from build123d import *

# Parameters (mm, degrees)
SKETCH1_W           = 119.2
SKETCH1_H           = 65.04
BOSS_EXTRUDE1_DEPTH = 2
SKETCH2_W           = 80
SKETCH2_H           = 2
SKETCH2_W_2         = 59.6
SKETCH2_H_2         = 2.5
BOSS_EXTRUDE2_DEPTH = 10
FILLET1_R           = 1
SKETCH3_W           = 80
SKETCH3_H           = 2
CUT_EXTRUDE1_DEPTH  = 7
SKETCH4_W           = 80
SKETCH4_H           = 2.5
SKETCH4_W_2         = 8
BOSS_EXTRUDE3_DEPTH = 10
FILLET2_R           = 1
FILLET3_R           = 1
CUT_EXTRUDE2_DEPTH  = 10
CUT_EXTRUDE3_DEPTH  = 10


with BuildPart() as part:
    # Sketch1 → Boss-Extrude1 (new body)
    with BuildSketch(Plane(origin=(0, 0, 0), x_dir=(1, 0, 0), z_dir=(0, 1, 0))):
        Rectangle(SKETCH1_W, SKETCH1_H)
    extrude(amount=BOSS_EXTRUDE1_DEPTH)

    # Sketch2 → Boss-Extrude2 (add)
    with BuildSketch(Plane(origin=(0, 2, 0), x_dir=(1, 0, 0), z_dir=(0, 1, 0))):
        with Locations((0, -9.48)):
            Rectangle(SKETCH2_W, SKETCH2_H)
        with Locations((0, -5.48)):
            Rectangle(SKETCH2_W, SKETCH2_H)
        with Locations((0, 28.27)):
            Rectangle(SKETCH2_W_2, SKETCH2_H_2)
    extrude(amount=BOSS_EXTRUDE2_DEPTH)

    # Fillet1
    fillet1_edges = [part.edges().sort_by_distance(p)[0] for p in [
        (40, 2, 9.48),
        (0, 2, 10.48),
        (-40, 2, 9.48),
        (40, 2, 5.48),
        (0, 2, 4.48),
        (-40, 2, 5.48),
        (-29.8, 2, -28.27),
        (29.8, 2, -28.27),
        (0, 2, -29.52),
    ]]
    fillet(fillet1_edges, radius=FILLET1_R)

    # Sketch3 → Cut-Extrude1 (cut)
    with BuildSketch(Plane(origin=(0, 12, 0), x_dir=(1, 0, 0), z_dir=(0, 1, 0))):
        with Locations((0, -5.48)):
            Rectangle(SKETCH3_W, SKETCH3_H)
        with Locations((0, -9.48)):
            Rectangle(SKETCH3_W, SKETCH3_H)
    extrude(amount=-CUT_EXTRUDE1_DEPTH, mode=Mode.SUBTRACT)

    # Sketch4 → Boss-Extrude3 (add)
    with BuildSketch(Plane(origin=(0, 2, 0), x_dir=(1, 0, 0), z_dir=(0, 1, 0))):
        with Locations((0, -28.77)):
            Rectangle(SKETCH4_W, SKETCH4_H)
        with Locations((52.6, -26.27)):
            Rectangle(SKETCH4_W_2, SKETCH4_H)
    boss_extrude3 = extrude(amount=BOSS_EXTRUDE3_DEPTH)

    # Fillet2
    fillet2_edges = [part.edges().sort_by_distance(p)[0] for p in [
        (-40, 2, 28.77),
        (48.6, 2, 26.27),
        (52.6, 2, 25.02),
        (40, 2, 28.77),
        (0, 2, 27.52),
    ]]
    fillet(fillet2_edges, radius=FILLET2_R)

    # Mirror1: Boss-Extrude3 across plane
    add(boss_extrude3.mirror(Plane.ZY))

    # Fillet3
    fillet3_edges = [part.edges().sort_by_distance(p)[0] for p in [
        (-48.6, 2, 26.27),
        (-52.6, 2, 25.02),
    ]]
    fillet(fillet3_edges, radius=FILLET3_R)

    # Sketch5 → Cut-Extrude2 (cut)
    with BuildSketch(Plane(origin=(0, 2, 0), x_dir=(1, 0, 0), z_dir=(0, 1, 0))):
        with BuildLine():
            Line((46.6, 22.52), (6.311514948, 22.52))
            Line((6.311514948, 22.52), (-46.6, 22.52))
            ThreePointArc((-46.6, 22.52), (-48.721320344, 21.641320344), (-49.6, 19.52))
            Line((-49.6, 19.52), (-49.6, 3.52))
            ThreePointArc((-49.6, 3.52), (-48.721320344, 1.398679656), (-46.6, 0.52))
            Line((-46.6, 0.52), (46.6, 0.52))
            ThreePointArc((46.6, 0.52), (48.721320344, 1.398679656), (49.6, 3.52))
            Line((49.6, 3.52), (49.6, 19.52))
            ThreePointArc((49.6, 19.52), (48.721320344, 21.641320344), (46.6, 22.52))
        make_face()
    extrude(amount=-CUT_EXTRUDE2_DEPTH, mode=Mode.SUBTRACT)

    # Sketch6 → Cut-Extrude3 (cut)
    with BuildSketch(Plane(origin=(0, 2, 0), x_dir=(1, 0, 0), z_dir=(0, 1, 0))):
        with BuildLine():
            Line((54.014213562, -5.94084617), (52.045315698, -3.971948306))
            ThreePointArc((52.045315698, -3.971948306), (51.396469, -3.538402803), (50.631102135, -3.386161868))
            Line((50.631102135, -3.386161868), (46.32782558, -3.386161868))
            ThreePointArc((46.32782558, -3.386161868), (44.913612017, -3.971948306), (44.32782558, -5.386161868))
            Line((44.32782558, -5.386161868), (44.32782558, -20.397912268))
            ThreePointArc((44.32782558, -20.397912268), (44.913612017, -21.812125831), (46.32782558, -22.397912268))
            Line((46.32782558, -22.397912268), (52.6, -22.397912268))
            ThreePointArc((52.6, -22.397912268), (54.014213562, -21.812125831), (54.6, -20.397912268))
            Line((54.6, -20.397912268), (54.6, -7.355059733))
            ThreePointArc((54.6, -7.355059733), (54.447759065, -6.589692868), (54.014213562, -5.94084617))
        make_face()
        with BuildLine():
            Line((39.82782558, -13.44932419), (24.210760832, -13.44932419))
            ThreePointArc((24.210760832, -13.44932419), (23.503654051, -13.742217409), (23.210760832, -14.44932419))
            Line((23.210760832, -14.44932419), (23.210760832, -23.393622011))
            ThreePointArc((23.210760832, -23.393622011), (23.650100661, -24.454282183), (24.710760832, -24.893622011))
            Line((24.710760832, -24.893622011), (39.32782558, -24.893622011))
            ThreePointArc((39.32782558, -24.893622011), (40.388485752, -24.454282183), (40.82782558, -23.393622011))
            Line((40.82782558, -23.393622011), (40.82782558, -14.44932419))
            ThreePointArc((40.82782558, -14.44932419), (40.534932361, -13.742217409), (39.82782558, -13.44932419))
        make_face()
        with BuildLine():
            Line((4.043952302, -24.893622011), (19.660852384, -24.893622011))
            ThreePointArc((19.660852384, -24.893622011), (20.367959165, -24.600728792), (20.660852384, -23.893622011))
            Line((20.660852384, -23.893622011), (20.660852384, -14.321364431))
            ThreePointArc((20.660852384, -14.321364431), (20.221512556, -13.260704259), (19.160852384, -12.821364431))
            Line((19.160852384, -12.821364431), (4.543952302, -12.821364431))
            ThreePointArc((4.543952302, -12.821364431), (3.48329213, -13.260704259), (3.043952302, -14.321364431))
            Line((3.043952302, -14.321364431), (3.043952302, -23.893622011))
            ThreePointArc((3.043952302, -23.893622011), (3.336845521, -24.600728792), (4.043952302, -24.893622011))
        make_face()
        with BuildLine():
            Line((-4.043952302, -24.893622011), (-19.660852384, -24.893622011))
            ThreePointArc((-19.660852384, -24.893622011), (-20.367959165, -24.600728792), (-20.660852384, -23.893622011))
            Line((-20.660852384, -23.893622011), (-20.660852384, -14.321364431))
            ThreePointArc((-20.660852384, -14.321364431), (-20.221512556, -13.260704259), (-19.160852384, -12.821364431))
            Line((-19.160852384, -12.821364431), (-4.543952302, -12.821364431))
            ThreePointArc((-4.543952302, -12.821364431), (-3.48329213, -13.260704259), (-3.043952302, -14.321364431))
            Line((-3.043952302, -14.321364431), (-3.043952302, -23.893622011))
            ThreePointArc((-3.043952302, -23.893622011), (-3.336845521, -24.600728792), (-4.043952302, -24.893622011))
        make_face()
        with BuildLine():
            Line((-39.32782558, -24.893622011), (-24.710760832, -24.893622011))
            ThreePointArc((-24.710760832, -24.893622011), (-23.650100661, -24.454282183), (-23.210760832, -23.393622011))
            Line((-23.210760832, -23.393622011), (-23.210760832, -14.44932419))
            ThreePointArc((-23.210760832, -14.44932419), (-23.503654051, -13.742217409), (-24.210760832, -13.44932419))
            Line((-24.210760832, -13.44932419), (-39.82782558, -13.44932419))
            ThreePointArc((-39.82782558, -13.44932419), (-40.534932361, -13.742217409), (-40.82782558, -14.44932419))
            Line((-40.82782558, -14.44932419), (-40.82782558, -23.393622011))
            ThreePointArc((-40.82782558, -23.393622011), (-40.388485752, -24.454282183), (-39.32782558, -24.893622011))
        make_face()
        with BuildLine():
            Line((-44.32782558, -5.386161868), (-44.32782558, -20.397912268))
            ThreePointArc((-44.32782558, -20.397912268), (-44.913612017, -21.812125831), (-46.32782558, -22.397912268))
            Line((-46.32782558, -22.397912268), (-52.6, -22.397912268))
            ThreePointArc((-52.6, -22.397912268), (-54.014213562, -21.812125831), (-54.6, -20.397912268))
            Line((-54.6, -20.397912268), (-54.6, -7.355059733))
            ThreePointArc((-54.6, -7.355059733), (-54.447759065, -6.589692868), (-54.014213562, -5.94084617))
            Line((-54.014213562, -5.94084617), (-52.045315698, -3.971948306))
            ThreePointArc((-52.045315698, -3.971948306), (-51.396469, -3.538402803), (-50.631102135, -3.386161868))
            Line((-50.631102135, -3.386161868), (-46.32782558, -3.386161868))
            ThreePointArc((-46.32782558, -3.386161868), (-44.913612017, -3.971948306), (-44.32782558, -5.386161868))
        make_face()
    extrude(amount=-CUT_EXTRUDE3_DEPTH, mode=Mode.SUBTRACT)


solid = part.part
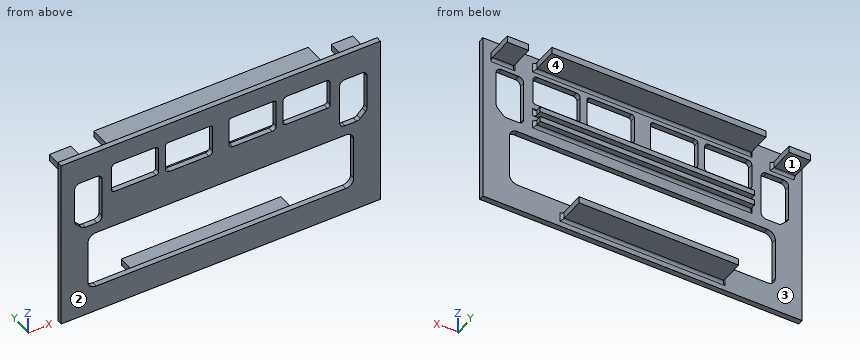
Verification items for the finished model (mm, model axes). Face numbers are marked on the shaded views. Give positions to 0.01 mm unless a question says otherwise; leave off trailing zeros. Loops run counter-clockwise (first coordinate to the right, second up) from the corner with the lowest first, then second, coordinate; pieces in that order, holes last. Notation, with made-up numbers: (33.5, 29) - (70.5, 29) arc R26 cw to (70.5, 55) - close; hole circle Ø4 at (25.25, 35.5). An arc over 180 degrees is marked (long way). Write item = value, one per line. Start each with the question number.
Q1. Thickness scan on line 1 (Z direction, x = -19.5, y = 3.25); line 2 (X direction, y = 8.5, z = 25.5); line 3 (Z direction, x = 15.5, y = 10.5). Record the ranges inside material, lowest first.
Q2. Cross-section at D-D, the plane z = -9. Enter the section's corners in (x, y).
Q3. Mould release check, pull along Z, two halves, no side actions. Record for the marked faces 1, 2, 3 and 4: released by +Z, released by -Z, zero draft, split by the parting line, or undercut.
Q4. Cross-section at C-C, the plane z = 18.5. Enter the section's corners in (x, y).
Q5. Cross-section at A-A, the plane x = 34. Enter the section's corners in (y, z).
Q6. Depth check by flat-ended pin: P1, Ø1, axis at y = 3.5, z = 9.5, coming from the -X side; P2, Ø3, axis at y = 7, z = 26.5, coming from the +X side; P3, Ø8, axis at x = 40, z = -17, coming from the +Y side; P4, Ø2, axis at x = -4.5, y = 5, coming from the +Z side. Enter the tip coordinate at first touch or a pass-through.
Q7. Cross-section at B-B, the plane y = 7.5. Enter the section's corners in (x, z), and give its area (3 significant figures).
Answer key:
q1.line_1 = -29.52 to -27.02, 4.48 to 6.48, 8.48 to 10.48, 27.52 to 30.02
q1.line_2 = -56.6 to -48.6, 48.6 to 56.6
q1.line_3 = -29.52 to -27.02, 27.52 to 30.02
q2.outline = (-59.6, 0) - (-49.6, 0) - (-49.6, 2) - (-59.6, 2) - close; (49.6, 0) - (59.6, 0) - (59.6, 2) - (49.6, 2) - close
q3.face_1 = released by -Z
q3.face_2 = zero draft
q3.face_3 = undercut
q3.face_4 = undercut
q4.outline = (-59.6, 0) - (-54.6, 0) - (-54.6, 2) - (-59.6, 2) - close; (-44.33, 0) - (-40.83, 0) - (-40.83, 2) - (-44.33, 2) - close; (-23.21, 0) - (-20.66, 0) - (-20.66, 2) - (-23.21, 2) - close; (-3.04, 0) - (3.04, 0) - (3.04, 2) - (-3.04, 2) - close; (20.66, 0) - (23.21, 0) - (23.21, 2) - (20.66, 2) - close; (40.83, 0) - (44.33, 0) - (44.33, 2) - (40.83, 2) - close; (54.6, 0) - (59.6, 0) - (59.6, 2) - (54.6, 2) - close
q5.outline = (0, -32.52) - (2, -32.52) - (2, -22.52) - (0, -22.52) - close; (0, -0.52) - (2, -0.52) - (2, 3.48) arc R1 cw to (3, 4.48) - (5, 4.48) - (5, 6.48) - (2, 6.48) - (2, 8.48) - (5, 8.48) - (5, 10.48) - (3, 10.48) arc R1 cw to (2, 11.48) - (2, 13.45) - (0, 13.45) - close; (0, 24.89) - (2, 24.89) - (2, 26.52) arc R1 cw to (3, 27.52) - (12, 27.52) - (12, 30.02) - (2, 30.02) - (2, 32.52) - (0, 32.52) - close
q6.P1 = -40
q6.P2 = 56.6
q6.P3 = through
q6.P4 = 30.02
q7.outline = (-56.6, 25.02) - (-48.6, 25.02) - (-48.6, 27.52) - (-56.6, 27.52) - close; (-40, 27.52) - (40, 27.52) - (40, 30.02) - (-40, 30.02) - close; (-29.8, -29.52) - (29.8, -29.52) - (29.8, -27.02) - (-29.8, -27.02) - close; (48.6, 25.02) - (56.6, 25.02) - (56.6, 27.52) - (48.6, 27.52) - close
q7.area = 389 mm^2
